Here's the drawing with two shaded views (mm, measured from the low corner). I have some questions. A direction names the side the tool comes from. Round coordinates to 2 decimals unless told otherwise and drop trailing zeros. Loops run counter-clockwise (first coordinate to the right, second up) from the corner with the lowest first, then second, coordinate; pieces in that order, holes last. Notation, with made-up numbers: M 76,67.5 L 94,67.5 A11 ccw 94,79.5 Z; hole C 6.5,0.5 d3. An arc over 180 degrees is marked long. Answer as a JSON object with one key per item and string values.
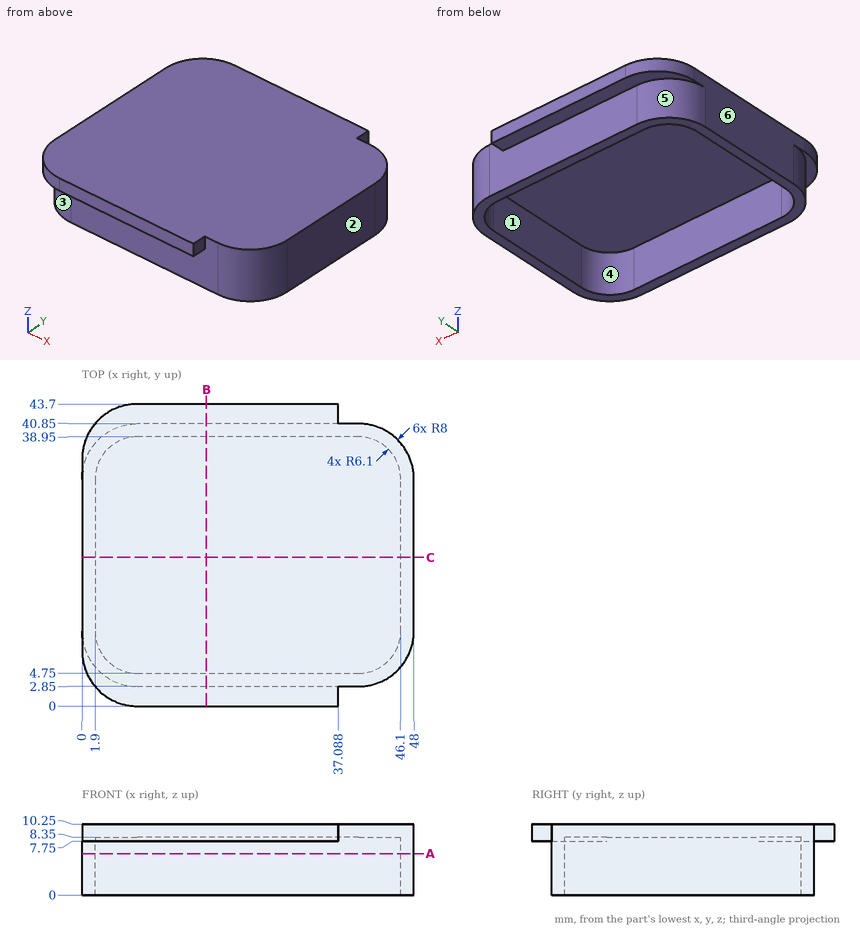
Item 1: I want a section at C-C on y = 21.5. List the corners of the cut face in (x, z) for me.
Solution:
{"outline": "M 0,0 L 1.9,0 L 1.9,8.35 L 46.1,8.35 L 46.1,0 L 48,0 L 48,10.25 L 0,10.25 Z"}
Item 2: For the marked faces 1 and 2, which set-ups out of +Z, -Z, +X, -X, +Y, -Y let a thin tool reach every point of the face, with its end or its side?
Solution:
{"face 1": "-Z", "face 2": "+Z, -Z, +X, +Y, -Y"}
Item 3: If I drill on L1, parallel to Y at x = 22.5, z = 4.5; L2, parallel to X at y = 27.5, z = 6; L3, parallel to Z at x = 8.5, y = 18, over which ranges is the centre line in solid material (lowest first)? Write a range as from..to.
Solution:
{"L1": "y = 2.85..4.75, 38.95..40.85", "L2": "x = 0..1.9, 46.1..48", "L3": "z = 8.35..10.25"}
Item 4: I want a section at A-A on z = 6. List the corners of the cut face in (x, y) for me.
Solution:
{"outline": "M 0,10.85 A8 ccw 8,2.85 L 40,2.85 A8 ccw 48,10.85 L 48,32.85 A8 ccw 40,40.85 L 8,40.85 A8 ccw 0,32.85 Z; hole M 1.9,10.85 A6.1 ccw 8,4.75 L 40,4.75 A6.1 ccw 46.1,10.85 L 46.1,32.85 A6.1 ccw 40,38.95 L 8,38.95 A6.1 ccw 1.9,32.85 Z"}
Item 5: I want a section at B-B on x = 18. List the corners of the cut face in (y, z) for me.
Solution:
{"outline": "M 0,7.75 L 2.85,7.75 L 2.85,0 L 4.75,0 L 4.75,8.35 L 38.95,8.35 L 38.95,0 L 40.85,0 L 40.85,7.75 L 43.7,7.75 L 43.7,10.25 L 0,10.25 Z"}
Item 6: For P1, Ø3, axis at x = 24.5, z = 4, coming from the +Y side; P2, Ø3, axis at x = 11.5, y = 19, coming from the -Z side; P3, Ø1.5, axis at y = 4.5, z = 5.5, coming from the -X side, each with a flat end and sliding along its axis, tell me the tip position at first contact or that it passes through.
Solution:
{"P1": "stops at y = 40.85", "P2": "stops at z = 8.35", "P3": "stops at x = 2.29"}
Item 7: We'd pull the mould along Y, two halves only. Please class the marked faces 3, 4, 5 and 6: +Y half, -Y half, draft (parallel to the pull), parting line (faces both ways), or undercut.
Solution:
{"face 3": "-Y half", "face 4": "undercut", "face 5": "+Y half", "face 6": "draft"}
